from build123d import *

# Parameters (mm, degrees)
F1_DEPTH = 14
F2_R     = 2.75
F3_DEPTH = 6
F4_SIZE  = 0.5


with BuildPart() as f1:
    # F0 (on Front) → F1 (new body)
    with BuildSketch(Plane.XZ):
        with BuildLine():
            Line((-21, -10.4), (-21, -16.4))
            Line((-21, -16.4), (21, -16.4))
            Line((21, -16.4), (21, -10.4))
            Line((21, -10.4), (9, -10.4))
            Line((9, -10.4), (9, 16.4))
            Line((9, 16.4), (0.4, 16.4))
            Line((0.4, 16.4), (0.4, 7.5799497484))
            ThreePointArc((0.4, 7.5799497484), (2.9664793948, 6.283281573), (4, 3.6))
            ThreePointArc((4, 3.6), (-2.683281573, 0.6335206052), (-0.4, 7.5799497484))
            Line((-0.4, 7.5799497484), (-0.4, 16.4))
            Line((-0.4, 16.4), (-9, 16.4))
            Line((-9, 16.4), (-9, -10.4))
            Line((-9, -10.4), (-21, -10.4))
        make_face()
    extrude(amount=F1_DEPTH)

    # F2 (on face) → F3 (cut)
    with BuildSketch(Plane(origin=(0, 0, -16.4), x_dir=(1, 0, 0), z_dir=(0, 0, -1))):
        with Locations((-16, 7)):
            Circle(F2_R)
        with Locations((16, 7)):
            Circle(F2_R)
    extrude(amount=-F3_DEPTH, mode=Mode.SUBTRACT)

    # F4
    f4_edges = [f1.edges().sort_by_distance(p)[0] for p in [
        (9, -7, 16.4),
        (-4.7, -14, 16.4),
        (-4.7, 0, 16.4),
        (-9, -7, 16.4),
        (9, -14, 3),
        (9, 0, 3),
        (15, 0, -10.4),
        (15, -14, -10.4),
        (21, -7, -10.4),
        (21, -14, -13.4),
        (21, 0, -13.4),
        (-9, -14, 3),
        (-15, -14, -10.4),
        (-21, -14, -13.4),
        (-21, -7, -10.4),
        (-9, 0, 3),
        (-15, 0, -10.4),
        (-21, 0, -13.4),
        (4.7, 0, 16.4),
        (4.7, -14, 16.4),
    ]]
    chamfer(f4_edges, length=F4_SIZE)


solid = f1.part
CAD build for the part. Positions are in the model's coordinates, mm. A direction names the side the tool comes from. Coordinates: 2 decimals unless noted, no trailing zeros. Write each loop counter-clockwise with the first axis right and the second up, starting at its lowest first coordinate (ties: lowest second). Pieces come first, ordered by that corner, then holes. Notation, with made-up numbers: M 78.25,43.5 L 134.25,43.5 A6 ccw 134.25,47.5 Z; hole C 86,84.25 d2. An arc over 180 degrees is marked long. Answer as a JSON object with one key per item and string values. Group by question number.
1) Pin check, flat tips, straight feed: pin 1 Ø6 at (x, y) = (14, -6.5) entering from +Z; pin 2 Ø6 at (y, z) = (-6, 12) entering from -X; pin 3 Ø3 at (y, z) = (-1.5, 8) entering from +X. Stop position of each tip, or through.
2) Saw through at B-B (y = -7). Write the cut outline in (x, z).
3) Saw through at A-A (x = 16). Write the cut outline in (y, z), plus the area to 4 significant figures.
4) Wall check: line 1 (X direction, y = -7, z = -11.55); line 2 (Y direction, x = 16, z = -14.4); line 3 (X direction, y = -11, z = 10). Give the ranges that are in metal, low to high. Write a range as from..to.
5) Saw through at D-D (z = 14.5). Write the cut outline in (x, y).
6) Saw through at C-C (z = -11.5). Write the cut outline in (x, y), plus the area to 3 significant figures.
7) Tool access for faces 1 (the face through (-0.4, -7, 12)), 2 (the face through (13.818, -5.327, -13.442)), 3 (the face through (-9, -7, 3)), 4 (the face through (5, -7, 16.4)), 5 (the face through (12, -7, -10.4)): list every direction of +Z, -Z, +X, -X, +Y, -Y with a clear straight run to the whole face (end or side of a thin tool).
8) Mould opens along X. For faces 6 (the face through (9, -7, 3)), 7 (the face through (0.4, -7, 12)), 8 (the face through (0, -7, -16.4)) say: +X half, -X half, draft (parallel to the pull), parting line (faces both ways), or undercut.
Values follow:
{
 "1": {"pin 1": "stops at z = -10.4", "pin 2": "stops at x = -9", "pin 3": "stops at x = 9"},
 "2": {"outline": "M -21,-16.4 L -18.75,-16.4 L -18.75,-10.4 L -20.5,-10.4 L -21,-10.9 Z; M -13.25,-16.4 L 13.25,-16.4 L 13.25,-10.4 L 9,-10.4 L 9,15.9 L 8.5,16.4 L 0.4,16.4 L 0.4,7.58 A4 cw long -0.4,7.58 L -0.4,16.4 L -8.5,16.4 L -9,15.9 L -9,-10.4 L -13.25,-10.4 Z; M 18.75,-16.4 L 21,-16.4 L 21,-10.9 L 20.5,-10.4 L 18.75,-10.4 Z"},
 "3": {"outline": "M -14,-16.4 L -9.75,-16.4 L -9.75,-10.4 L -13.5,-10.4 L -14,-10.9 Z; M -4.25,-16.4 L 0,-16.4 L 0,-10.9 L -0.5,-10.4 L -4.25,-10.4 Z", "area": "50.75 mm2"},
 "4": {"line 1": "x = -21..-18.75, -13.25..13.25, 18.75..21", "line 2": "y = -14..-9.75, -4.25..0", "line 3": "x = -9..-0.4, 0.4..9"},
 "5": {"outline": "M -9,-13.5 L -8.5,-14 L -0.4,-14 L -0.4,0 L -8.5,0 L -9,-0.5 Z; M 0.4,-14 L 8.5,-14 L 9,-13.5 L 9,-0.5 L 8.5,0 L 0.4,0 Z"},
 "6": {"outline": "M -21,-13.5 L -20.5,-14 L 20.5,-14 L 21,-13.5 L 21,-0.5 L 20.5,0 L -20.5,0 L -21,-0.5 Z; hole C -16,-7 d5.5; hole C 16,-7 d5.5", "area": "540 mm2"},
 "7": {"face 1": "+Z, +Y, -Y", "face 2": "+Z, -Z", "face 3": "+Z, -X, +Y, -Y", "face 4": "+Z, +X, -X, +Y, -Y", "face 5": "+Z, +X, +Y, -Y"},
 "8": {"face 6": "+X half", "face 7": "undercut", "face 8": "draft"}
}
